Design review of the part built by this model. Coordinates are the model's own, in mm. A direction names the side the tool comes from. Coordinates: 2 decimals unless noted, no trailing zeros. Write each loop counter-clockwise with the first axis right and the second up, starting at its lowest first coordinate (ties: lowest second). Pieces come first, ordered by that corner, then holes. Notation, with made-up numbers: (-34, 55.5) - (-22, 55.5) arc R30 cw to (-22, 90.5) - close; hole circle Ø9 at (68.25, -23). An arc over 180 degrees is marked (long way). Answer as a JSON object with one key per item and string values.
```python
from build123d import *

# Parameters (mm, degrees)
ESQUISSE1_W                                      = 78
ESQUISSE1_H                                      = 64
ESQUISSE1_R                                      = 1.5
BOSS_EXTRU_1_DEPTH                               = 8
FRAISAGE_POUR_VIS_T_TE_FRAIS_E_M31_D             = 3.4
FRAISAGE_POUR_VIS_T_TE_FRAIS_E_M31_DEPTH         = 8
FRAISAGE_POUR_VIS_T_TE_FRAIS_E_M31_CSINK_D       = 6.3
FRAISAGE_POUR_VIS_T_TE_FRAIS_E_M31_CSINK_ANGLE   = 90
ESQUISSE4_W                                      = 59
ESQUISSE4_H                                      = 47
BOSS_EXTRU_2_DEPTH                               = 20
ENL_V_START                                      = -27.764118658
ENL_V_MAT_EXTRU_1_OUTLINE_W                      = 62
ENL_V_MAT_EXTRU_1_OUTLINE_H                      = 50
ENL_V_MAT_EXTRU_1_DEPTH                          = 1.24955815
ESQUISSE14_W                                     = 78
ESQUISSE14_H                                     = 64
ESQUISSE14_R                                     = 1
BOSS_EXTRU_4_DEPTH                               = 2.5
FRAISAGE_POUR_VIS_T_TE_FRAIS_E_M2_53_D           = 2.9
FRAISAGE_POUR_VIS_T_TE_FRAIS_E_M2_53_DEPTH       = 2.5
FRAISAGE_POUR_VIS_T_TE_FRAIS_E_M2_53_CSINK_D     = 5.5
FRAISAGE_POUR_VIS_T_TE_FRAIS_E_M2_53_CSINK_ANGLE = 90
FRAISAGE_POUR_VIS_T_TE_FRAIS_E_M2_53_TIP         = 0.871247898
ENL_V_MAT_EXTRU_2_REACH                          = 108.208
ESQUISSE20_W                                     = 40
ESQUISSE20_H                                     = 10
CONG_1_R                                         = 3


# Read off the part's stored shape, not the designer's step: Enlèv. mat.-Extru.1
with BuildPart() as part:
    # Esquisse1 → Boss.-Extru.1 (new body)
    with BuildSketch(Plane.XY):
        with Locations((39, 32)):
            Rectangle(ESQUISSE1_W, ESQUISSE1_H)
        with Locations((4, 60)):
            Circle(ESQUISSE1_R, mode=Mode.SUBTRACT)
        with Locations((4, 4)):
            Circle(ESQUISSE1_R, mode=Mode.SUBTRACT)
        with Locations((74, 12)):
            Circle(ESQUISSE1_R, mode=Mode.SUBTRACT)
        with Locations((74, 52)):
            Circle(ESQUISSE1_R, mode=Mode.SUBTRACT)
    extrude(amount=BOSS_EXTRU_1_DEPTH)

    # Fraisage pour vis à tête fraisée M31
    with Locations(Plane.XY.offset(8)):
        with Locations((4, 60), (4, 4), (74, 12), (74, 52)):
            CounterSinkHole(FRAISAGE_POUR_VIS_T_TE_FRAIS_E_M31_D / 2, FRAISAGE_POUR_VIS_T_TE_FRAIS_E_M31_CSINK_D / 2, depth=FRAISAGE_POUR_VIS_T_TE_FRAIS_E_M31_DEPTH, counter_sink_angle=FRAISAGE_POUR_VIS_T_TE_FRAIS_E_M31_CSINK_ANGLE)

    # Esquisse4 → Boss.-Extru.2 (add)
    with BuildSketch(Plane.XY.offset(8)):
        with Locations((39, 32)):
            Rectangle(ESQUISSE4_W, ESQUISSE4_H)
    extrude(amount=BOSS_EXTRU_2_DEPTH)

    # Enlèv. mat.-Extru.1 outline → Enlèv. mat.-Extru.1 (cut)
    with BuildSketch(Plane(origin=(0, 0, 0), x_dir=(1, 0, 0), z_dir=(0, 0.026586343635431896, -0.9996465206922389)).offset(ENL_V_START)):
        with Locations((39, -33)):
            Rectangle(ENL_V_MAT_EXTRU_1_OUTLINE_W, ENL_V_MAT_EXTRU_1_OUTLINE_H)
    extrude(amount=ENL_V_MAT_EXTRU_1_DEPTH, mode=Mode.SUBTRACT)

    # Esquisse14 → Boss.-Extru.4 (add)
    with BuildSketch(Plane(origin=(0, 17.262764885, 26.983052258), x_dir=(1, 0, 0), z_dir=(0, 0.026586343635431917, -0.9996465206922389))):
        with Locations((40, -14.216024519)):
            Rectangle(ESQUISSE14_W, ESQUISSE14_H)
        with Locations(Location((5, 13.783975481, 0), (0, 0, 270))):
            Circle(ESQUISSE14_R, mode=Mode.SUBTRACT)
        with Locations(Location((5, -42.216024519, 0), (0, 0, 270))):
            Circle(ESQUISSE14_R, mode=Mode.SUBTRACT)
        with Locations(Location((75, -34.216024519, 0), (0, 0, 270))):
            Circle(ESQUISSE14_R, mode=Mode.SUBTRACT)
        with Locations(Location((75, 5.783975481, 0), (0, 0, 270))):
            Circle(ESQUISSE14_R, mode=Mode.SUBTRACT)
    extrude(amount=-BOSS_EXTRU_4_DEPTH)

    # Fraisage pour vis à tête fraisée M2.53
    with Locations(Plane(origin=(0, -0.704925217, 26.505188159), x_dir=(-1, 0, 0), z_dir=(0, 0.02658634363543186, -0.9996465206922389))):
        with Locations((-5, 60.190068073), (-5, 4.190068073), (-75, 12.190068073), (-75, 52.190068073)):
            CounterSinkHole(FRAISAGE_POUR_VIS_T_TE_FRAIS_E_M2_53_D / 2, FRAISAGE_POUR_VIS_T_TE_FRAIS_E_M2_53_CSINK_D / 2, depth=FRAISAGE_POUR_VIS_T_TE_FRAIS_E_M2_53_DEPTH, counter_sink_angle=FRAISAGE_POUR_VIS_T_TE_FRAIS_E_M2_53_CSINK_ANGLE)
            with Locations((0, 0, -(FRAISAGE_POUR_VIS_T_TE_FRAIS_E_M2_53_DEPTH + FRAISAGE_POUR_VIS_T_TE_FRAIS_E_M2_53_TIP / 2))):  # 118° drill point
                Cone(0, FRAISAGE_POUR_VIS_T_TE_FRAIS_E_M2_53_D / 2, FRAISAGE_POUR_VIS_T_TE_FRAIS_E_M2_53_TIP, mode=Mode.SUBTRACT)

    # Enlèv. mat.-Extru.2: up to this plane
    enl_v_mat_extru_2_end = Plane(origin=(0, -0.771391076, 29.004304461), z_dir=(0, -0.026586343635431952, 0.9996465206922389))
    # Esquisse20 → Enlèv. mat.-Extru.2 (cut, up to the surface)
    with BuildSketch(Plane(origin=(0, 0, 0), x_dir=(-1, 0, 0), z_dir=(0, 0, -1)), mode=Mode.PRIVATE) as enl_v_mat_extru_2_sk1:
        with Locations((-35, 3.418609812)):
            Rectangle(ESQUISSE20_W, ESQUISSE20_H)
    enl_v_mat_extru_2_tool1 = split(extrude(enl_v_mat_extru_2_sk1.sketch, amount=-ENL_V_MAT_EXTRU_2_REACH, mode=Mode.PRIVATE), bisect_by=enl_v_mat_extru_2_end, keep=Keep.BOTH, mode=Mode.PRIVATE)
    add(enl_v_mat_extru_2_tool1.solids().sort_by_distance((35, 3.41861, 0))[0], mode=Mode.SUBTRACT)

    # Congé1
    cong_1_edges = [part.edges().sort_by_distance(p)[0] for p in [
        (15, -0.548157258, 27.759799525),
        (55, -0.548157258, 27.759799525),
        (55, 8.418609812, 4),
        (55, 8.418609812, 27.998277373),
        (55, 0, 4),
        (15, 0, 4),
        (15, 8.418609812, 4),
        (15, 8.418609812, 27.998277373),
    ]]
    fillet(cong_1_edges, radius=CONG_1_R)


solid = part.part
```
(1) Take a section at B-B, the plane x = 59. Write out the cut boundary in (y, z), and give its area (3 significant figures).
Solved:
{"outline": "(-0.58, 29.01) - (-0.51, 26.51) - (8.5, 26.75) - (8.5, 8) - (0, 8) - (0, 0) - (64, 0) - (64, 8) - (55.5, 8) - (55.5, 28) - (63.46, 28.21) - (63.4, 30.71) - close", "area": "1,580 mm^2"}
(2) Take a section at D-D, the plane z = 17. Write out the cut boundary in (x, y).
Solved:
{"outline": "(9.5, 8.5) - (68.5, 8.5) - (68.5, 55.5) - (9.5, 55.5) - close"}
(3) Tool access review of faces 1 (the face through (55, 4, 28)), 2 (the face through (1, 32, 29)), 3 (the face through (75.7, 52.07, 3.23)), 4 (the face through (68, 0, 4)): name each direction out of +Z, -Z, +X, -X, +Y, -Y from which nothing blocks a thin tool from reaching the whole face with its end or side.
Solved:
{"face 1": "+Z, -Z, -Y", "face 2": "+Z, -X, +Y, -Y", "face 3": "-Z", "face 4": "-Z, +X, -X, -Y"}
(4) Take a section at C-C, the plane y = 45. Write out the cut boundary in (x, z).
Solved:
{"outline": "(0, 0) - (78, 0) - (78, 8) - (68.5, 8) - (68.5, 27.72) - (79, 27.72) - (79, 30.22) - (1, 30.22) - (1, 27.72) - (9.5, 27.72) - (9.5, 8) - (0, 8) - close"}
(5) The part is to be moulded in two halves that separate along Y. For faces 5 (the face through (35, 8.419, 4)), 6 (the face through (3.93, 60.39, 30.04)), 7 (the face through (15, 4, 28)), say which applies: pulls with the +Y half, pulls with the -Y half, needs draft (parallel to the pull), parting line crosses it, or undercut.
Solved:
{"face 5": "pulls with the -Y half", "face 6": "undercut", "face 7": "needs draft"}
(6) For pin 1 (2.5 mm diameter, centred on x = 4, y = 60, fed in from -Z); pin 2 (10 mm diameter, centred on x = 41.5, z = 20.5, fed in from +Y); pin 3 (1.5 mm diameter, centred on y = 47, z = 11.5, fed in from -X), all flat-tipped, find the tip position at first contact; note any pin that passes through.
Solved:
{"pin 1": "stops at z = 28.5", "pin 2": "stops at y = 55.5", "pin 3": "stops at x = 9.5"}
(7) Take a section at A-A, the plane z = 4. Write out the cut boundary in (x, y), and give its area (3 significant figures).
Solved:
{"outline": "(0, 0) - (12, 0) arc R3 ccw to (15, 3) - (15, 5.42) arc R3 cw to (18, 8.42) - (52, 8.42) arc R3 cw to (55, 5.42) - (55, 3) arc R3 ccw to (58, 0) - (78, 0) - (78, 64) - (0, 64) - close; hole circle Ø3.4 at (4, 4); hole circle Ø3.4 at (4, 60); hole circle Ø3.4 at (74, 12); hole circle Ø3.4 at (74, 52)", "area": "4,620 mm^2"}
(8) To check wall thickness, follow line 1 (Y direction, x = 4, z = 4.25); line 2 (X direction, y = 4, z = 2); line 3 (X direction, y = 12, z = 2.5). State the ranges of each line that lie inside material, in increasing order. Write a range as from..to.
Solved:
{"line 1": "y = 0..2.3, 5.7..58.3, 61.7..64", "line 2": "x = 0..2.3, 5.7..15, 55..78", "line 3": "x = 0..72.3, 75.7..78"}
